Geometry check sheet. Reference: the model listing, model coordinates, mm. Round coordinates to 2 decimals unless told otherwise and drop trailing zeros. Order: outer loops, then holes, each group sorted by start corner. A loop starts at its lowest first (then second) coordinate and runs counter-clockwise, first axis right, second up. Notation, with made-up numbers: (45.25, -12.75) - (71.25, -12.75) arc R29 ccw to (71.25, 12.25) - close; hole circle Ø3 at (84.25, -13.5). An arc over 180 degrees is marked (long way). Use a Markdown table: item, result. Add a question column.
(1) Section check A-A on y = -114. Record the boundary of the cut face in (x, z).
(2) Section check B-B on z = -849. Record the boundary of the cut face in (x, y), then the cut area to 3 significant figures.
(3) Gauge pin test, flat ends, axial feed: P1, Ø4.5, axis at x = 5, y = -5, coming from the -Z side; P2, Ø4, axis at x = 5, z = -751.5, coming from the -Y side; P3, Ø5, axis at x = -4, y = -384, coming from the +Z side. Record the tip position at first contact, or that the pin passes through.
(4) Thickness scan on line 1 along Y through (x, z) = (1, -733); line 2 along Z through (x, y) = (1.75, -229); line 3 along Y through (x, z) = (5, -0.7). Record the ranges inside material, lowest first. Write a range as [from, to].
Autodesk Inventor part; units mm, degrees
ref_plane "YZ Plane" through (0, 0, 0) normal (1, 0, 0) x (0, 1, 0)
ref_plane "XZ Plane" through (0, 0, 0) normal (0, 1, 0) x (-1, 0, 0)
ref_plane "XY Plane" through (0, 0, 0) normal (0, 0, 1) x (1, 0, 0)
sketch "Sketch1" plane through (0, 0, 0) normal (1, 0, 0) x (0, 1, 0)
  line L0 (0, 0) -> (-383, 0)
  line L1 (-383, 0) -> (-383, -1138)
  line L2 (-383, -1138) -> (0, -1138)
  line L3 (0, -1138) -> (0, 0)
  line L4 (-373, -1128) -> (-373, -10)
  line L5 (-373, -10) -> (-10, -10)
  line L6 (-10, -10) -> (-10, -1128)
  line L7 (-10, -1128) -> (-373, -1128)
  dimension "d0" = 383
  dimension "d1" = 1138
  dimension "d2" = 10
extrude "Extrusion1" add sketch "Sketch1" along normal blind 10
sketch "Sketch2" plane through (0, -383, 0) normal (0, 0, 1) x (1, 0, 0)
  line L0 (0, 383) -> (0, 0)
  line L1 (0, 0) -> (10, 0)
  line L2 (10, 383) -> (10, 0)
  line L3 (0, 383) -> (10, 383)
  line L4 (0, 0) -> (-3.182, -3.182)
  line L5 (0, 0) -> (4.5, 0) construction
  line L6 (0, 383) -> (0, 0)
  circle A0 centre (-3.182, -3.182) radius 5
  circle A1 centre (-3.182, -3.182) radius 4
  dimension "d5" = 4.5
  dimension "d6" = 135
  dimension "d7" = 1
  dimension "d10" = 10
extrude "Extrusion2" add sketch "Sketch2" against normal blind 35 contours A0 L1 L0 | L0 L1 A0
ref_plane "Work Plane1" through (0, 0, -569) normal (0, 0, 1) x (1, 0, 0)
mirror "Mirror1" about plane through (0, 0, -569) normal (0, 0, 1) of "Extrusion2"
fillet "Fillet1" [suppressed]
ref_plane "Work Plane2" through (0, -383, -1113) normal (0, 0, 1) x (1, 0, 0)
sketch "Sketch3" plane through (0, -383, -1113) normal (0, 0, 1) x (1, 0, 0)
  arc A0 (0, 0.6748) -> (0.6748, 0) centre (-3.182, -3.182) ccw
  circle A1 centre (-3.182, -3.182) radius 4
  line L0 (0.6748, 0) -> (10, 0)
  circle A2 centre (-3.182, -3.182) radius 5
  point P0 (0, 383)
  point P1 (0, 0.6748)
extrude "Extrusion3" cut sketch "Sketch3" against normal blind 15
sketch "Sketch4" plane through (0, 0, 0) normal (0, 0, 1) x (1, 0, 0)
  circle A0 centre (-3.182, -386.182) radius 4
  arc A1 (0, -382.3252) -> (0.6748, -383) centre (-3.182, -386.182) ccw
  circle A2 centre (-3.182, -386.182) radius 4
  line L0 (0.6748, -383) -> (10, -383)
  circle A3 centre (-3.182, -386.182) radius 5
  point P0 (0, 0)
  point P1 (0, -382.3252)
extrude "Extrusion4" cut sketch "Sketch4" against normal blind 10
sketch "Sketch5" plane through (0, -383, -35) normal (0, 0, -1) x (-1, 0, 0)
  circle A0 centre (3.182, -3.182) radius 4
  arc A1 (-0.6748, 0) -> (0, 0.6748) centre (3.182, -3.182) ccw
  circle A2 centre (3.182, -3.182) radius 5
  point P0 (0, 383)
  point P1 (0, 0.6748)
extrude "Extrusion5" cut sketch "Sketch5" against normal blind 10
sketch "Sketch6" plane through (0, 0, 0) normal (0, 0, 1) x (1, 0, 0)
  arc A0 (0.6748, -383) -> (0, -382.3252) centre (-3.182, -386.182) ccw
  line L0 (0.6748, -383) -> (10, -383)
  line L1 (10, 0) -> (10, -383)
  line L2 (0, 0) -> (10, 0)
  line L3 (0, 0) -> (0, -382.3252)
  line L4 (10, -383) -> (10, 0) construction
  line L5 (0, -10) -> (10, -10) construction
  line L6 (10, 0) -> (0, -10) construction
  line L7 (0, 0) -> (10, 0) construction
  line L8 (0, 0) -> (10, -10) construction
  circle A1 centre (5, -5) radius 2.5
  dimension "d19" = 5
extrude "Extrusion6" cut sketch "Sketch6" against normal blind 3 contours A1
sketch "Sketch7" plane through (5, -5, -3) normal (0, 0, 1) x (1, 0, 0)
  circle A0 centre (0, 0) radius 2.5
  circle A1 centre (0, 0) radius 7.5
  line L0 (13, -13) -> (-13, -13)
  line L1 (-13, -13) -> (-13, 13)
  line L2 (-13, 13) -> (13, 13)
  line L3 (13, 13) -> (13, -13)
  line L4 (13, -13) -> (-13, 13) construction
  line L5 (-13, -13) -> (13, 13) construction
  point P0 (-5, 5)
  dimension "d22" = 15
  dimension "d25" = 26
  dimension "d26" = 26
extrude "Extrusion7" [suppressed]
mirror "Mirror2" about plane through (0, 0, -569) normal (0, 0, 1) of "Extrusion6"
equation "\"d25\" = d26"
properties part number "porta1"
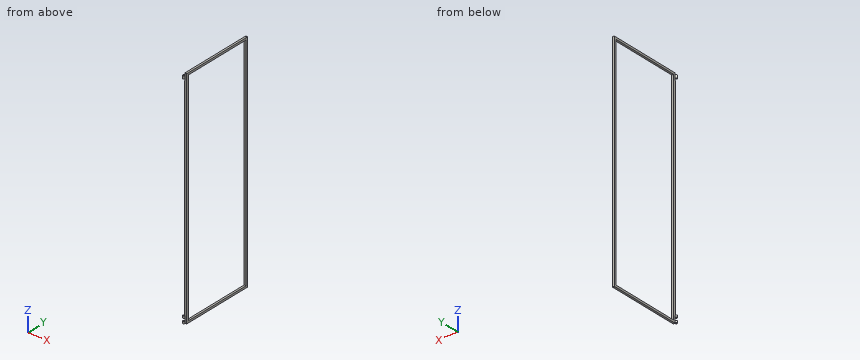
Check sheet entries:
| question | item | result |
|---|---|---|
| 1 | outline | (0, -1138) - (10, -1138) - (10, -1128) - (0, -1128) - close; (0, -10) - (10, -10) - (10, 0) - (0, 0) - close |
| 2 | outline | (0, -383) - (10, -383) - (10, -373) - (0, -373) - close; (0, -10) - (10, -10) - (10, 0) - (0, 0) - close |
| 2 | area | 200 mm2 |
| 3 | P1 | stops at z = -1135 |
| 3 | P2 | stops at y = -383 |
| 3 | P3 | stops at z = -10 |
| 4 | line 1 | y = [-383, -373], [-10, 0] |
| 4 | line 2 | z = [-1138, -1128], [-10, 0] |
| 4 | line 3 | y = [-383, -7.5], [-2.5, 0] |
